Part print with two shaded views. Sizes in mm from the minimum x, y, z corner. A direction names the side the tool comes from. Coordinates: 2 decimals unless noted, no trailing zeros. Order: outer loops, then holes, each group sorted by start corner. A loop starts at its lowest first (then second) coordinate and runs counter-clockwise, first axis right, second up. Notation, with made-up numbers: (-24.5, 11) - (-0.5, 11) arc R11 ccw to (-0.5, 21) - close; hole circle Ø5 at (5, 56.5). An arc over 180 degrees is marked (long way). Return JSON: item names as keys, results as strings.
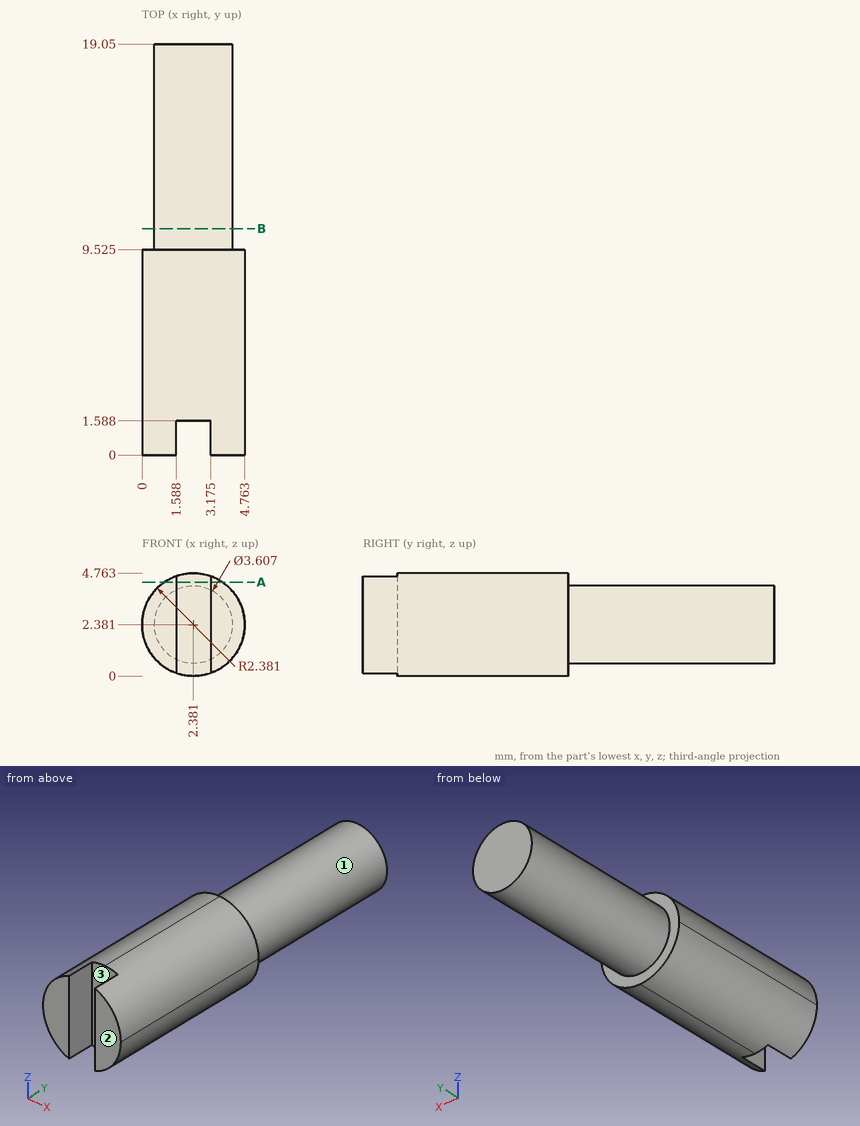
Item 1: Wall check: L1, parallel to X at y = 7.75, z = 2.45; L2, parallel to Y at x = 1.7, z = 1.4; L3, parallel to Y at x = 4.4, z = 2 (1 decimal). Give the ranges that are in metal, low to high. Write a range as [from, to].
Findings below:
{"L1": "x = [0, 4.76]", "L2": "y = [1.59, 19.05]", "L3": "y = [0, 9.5]"}
Item 2: Band-saw the part on A-A, the plane z = 4.35. List the corners of the cut face in (x, y) (1 decimal), then the cut area to 3 significant figures.
Findings below:
{"outline": "(1, 0) - (1.6, 0) - (1.6, 1.6) - (3.2, 1.6) - (3.2, 0) - (3.7, 0) - (3.7, 9.5) - (1, 9.5) - close", "area": "23.0 mm²"}
Item 3: Drop flat-ended pins along their axis: P1, Ø2, axis at y = 16.5, z = 1, coming from the -X side; P2, Ø1.5, axis at y = 3.5, z = 3.5, coming from the -X side; P3, Ø0.8, axis at y = 1, z = 3, coming from the +X side. Give the stop position or say it passes through.
Findings below:
{"P1": "stops at x = 0.62", "P2": "stops at x = 0.03", "P3": "stops at x = 4.75"}
Item 4: Which spindle directions (+Z, -Z, +X, -X, +Y, -Y) get a long thin tool onto all of the face, cutting with end or side? Do the marked faces 1, 2 and 3. Say none if no direction does.
Findings below:
{"face 1": "+Y", "face 2": "+Z, -Z, +X, -X, -Y", "face 3": "+Z, -Z, -Y"}
Item 5: Band-saw the part on B-B, the plane y = 10.5. List the corners of the cut face in (x, z).
Findings below:
{"outline": "circle Ø3.61 at (2.38, 2.38)"}
